Could you check a few things on this model? Use its own coordinates, in mm. A direction names the side the tool comes from. Coordinates: 2 decimals unless noted, no trailing zeros. Loops run counter-clockwise (first coordinate to the right, second up) from the corner with the lowest first, then second, coordinate; pieces in that order, holes last. Notation, with made-up numbers: (89, 2) -> (98, 2) arc R17 cw to (98, 18) -> close; hole circle Ø3 at (32.5, 65.25). An arc over 180 degrees is marked (long way). One line per question, with ' | ' between items.
Autodesk Inventor part; units mm, degrees
ref_plane "YZ Plane" through (0, 0, 0) normal (1, 0, 0) x (0, 1, 0)
ref_plane "XZ Plane" through (0, 0, 0) normal (0, 1, 0) x (-1, 0, 0)
ref_plane "XY Plane" through (0, 0, 0) normal (0, 0, 1) x (1, 0, 0)
sketch "Sketch1" plane through (0, 0, 0) normal (0, 0, 1) x (1, 0, 0)
  line L0 (-48, 48) -> (48, 48) construction
  line L1 (48, 48) -> (48, -48) construction
  line L2 (48, -48) -> (-48, -48) construction
  line L3 (-48, -48) -> (-48, 48) construction
  circle A0 centre (-45, 45) radius 2.25
  circle A1 centre (45, 45) radius 2.25
  line L4 (45, 45) -> (-45, 45) construction
  line L5 (-45, 45) -> (-45, -45) construction
  line L6 (-45, -45) -> (45, -45) construction
  line L7 (45, -45) -> (45, 45) construction
  circle A2 centre (45, -45) radius 2.25
  circle A3 centre (-45, -45) radius 2.25
  line L8 (-50.5, -50.5) -> (-42, -50.5)
  line L9 (-42, -50.5) -> (-42, -42)
  line L10 (-42, -42) -> (-50.5, -42)
  line L11 (-50.5, -42) -> (-50.5, -50.5)
  line L12 (0, 0) -> (-48, -48) construction
  line L13 (-33, 26.5) -> (33, 26.5)
  line L14 (33, 26.5) -> (33, -26.5)
  line L15 (33, -26.5) -> (-33, -26.5)
  line L16 (-33, -26.5) -> (-33, 26.5)
  line L17 (-2.4749, 2.4749) -> (2.4749, -2.4749)
  line L18 (2.4749, -2.4749) -> (-42.5251, -47.4749)
  line L19 (-42.5251, -47.4749) -> (-47.4749, -42.5251)
  line L20 (-47.4749, -42.5251) -> (-2.4749, 2.4749)
  line L21 (0, 0) -> (-45, -45) construction
  line L22 (31, 24.5) -> (-31, 24.5)
  line L23 (-31, 24.5) -> (-31, -24.5)
  line L24 (-31, -24.5) -> (31, -24.5)
  line L25 (31, -24.5) -> (31, 24.5)
  point P0 (0, 48)
  point P1 (48, 0)
  point P2 (33, 0)
  point P3 (0, 26.5)
  dimension "d0" = 96
  dimension "d1" = 96
  dimension "d2" = 4.5
  dimension "d3" = 4.5
  dimension "d4" = 3
  dimension "d5" = 4.5
  dimension "d6" = 4.5
  dimension "d9" = 3
  dimension "d10" = 3
  dimension "d11" = 66
  dimension "d12" = 53
  dimension "d13" = 7
  dimension "d14" = 0
  dimension "d23" = 5.5
  dimension "d24" = 5.5
  dimension "d25" = 2
extrude "Extrusion1" add sketch "Sketch1" along normal blind 1.5 contours L20 L24 L18 L15 | L15 L16 L13 L14 L18 L24 L25 L22 L23 L20 | L24 L23 L22 L25 L18 L17 L20 | L20 L17 L18 L24
extrude "Extrusion2" add sketch "Sketch1" along normal blind 1.5 contours A3 L19 | A3 L19 L20 L10 L9 L18 | A3 L19 L18 L9 L8 L11 L10 L20 | L20 L15 L18 L9 L10 | L20 L24 L18 L15 | L20 L17 L18 L24 picked at (-45.2318, -44.2867)
extrude "Extrusion3" cut sketch "Sketch1" along normal blind 10 contours A3 L19 | L19 A3
mirror "Mirror1" about plane through (0, 0, 0) normal (1, 0, 0) of "Extrusion2", "Extrusion3"
mirror "Mirror2" about plane through (0, 0, 0) normal (0, 1, 0) of "Extrusion2", "Extrusion3", "Mirror1"
extrude "Extrusion4" cut sketch "Sketch1" along normal blind 10 contours L24 L23 L22 L25 L18 L17 L20 | L20 L17 L18 L24
fillet "Fillet3" radius 3 4 edges at (31.4497, -26.5, 0.75) (31.4497, 26.5, 0.75) (-31.4497, 26.5, 0.75) (-31.4497, -26.5, 0.75)
fillet "Fillet4" radius 10 4 edges at (-21.5503, -26.5, 0.75) (21.5503, -26.5, 0.75) (21.5503, 26.5, 0.75) (-21.5503, 26.5, 0.75)
properties part number "BattHolder"
Q1. Imagine slicing it at C-C on x = 45. Write out the boundary of the cut face in (y, z), plus the area to 3 significant figures.
Values follow:
outline: (-50.5, 0) -> (-47.25, 0) -> (-47.25, 1.5) -> (-50.5, 1.5) -> close; (-42.75, 0) -> (-40.05, 0) -> (-40.05, 1.5) -> (-42.75, 1.5) -> close; (40.05, 0) -> (42.75, 0) -> (42.75, 1.5) -> (40.05, 1.5) -> close; (47.25, 0) -> (50.5, 0) -> (50.5, 1.5) -> (47.25, 1.5) -> close | area: 17.8 mm2
Q2. We'd pull the mould along X, two halves only. Please class faces 4 (the face through (21.286, -27.282, 0.76)), 5 (the face through (-40.5, -35.55, 0.74)), 6 (the face through (-21.286, 27.282, 0.76)), 7 (the face through (0, 26, 1.5)): released by +X, released by -X, zero draft, split by the parting line, or undercut.
Values follow:
face 4: undercut | face 5: released by -X | face 6: undercut | face 7: zero draft
Q3. Imagine slicing it at A-A on y = 2.5. Write out the boundary of the cut face in (x, z).
Values follow:
outline: (-33, 0) -> (-31, 0) -> (-31, 1.5) -> (-33, 1.5) -> close; (31, 0) -> (33, 0) -> (33, 1.5) -> (31, 1.5) -> close
Q4. For pin 1 (0.8 mm diameter, centred on x = -7.5, z = 0.5, fed in from -Y); pin 2 (0.8 mm diameter, centred on x = -1, z = 0.5, fed in from +Y), each with a flat end and sliding along its axis, tell me the tip position at first contact or that it passes through.
Values follow:
pin 1: stops at y = -26.5 | pin 2: stops at y = 26.5
Q5. For faces 1 (the face through (-40.32, 35.37, 0.74)), 2 (the face through (40.32, -35.37, 0.74)), 3 (the face through (-33.36, 38.31, 0.74)), which set-ups out of +Z, -Z, +X, -X, +Y, -Y let a thin tool reach every point of the face, with its end or its side?
Values follow:
face 1: +Z, -Z, -X | face 2: +Z, -Z, +X | face 3: +Z, -Z, +Y
Q6. Please list where these lines run through material, in increasing order: L1, parallel to Y at x = 10, z = 0.8; L2, parallel to Y at x = -45, z = 1.1. Write a range as [from, to].
Values follow:
L1: y = [-26.5, -24.5], [24.5, 26.5] | L2: y = [-50.5, -47.25], [-42.75, -40.05], [40.05, 42.75], [47.25, 50.5]
Q7. Imagine slicing it at B-B on x = -5. Write out the boundary of the cut face in (y, z), plus the area to 3 significant figures.
Values follow:
outline: (-26.5, 0) -> (-24.5, 0) -> (-24.5, 1.5) -> (-26.5, 1.5) -> close; (24.5, 0) -> (26.5, 0) -> (26.5, 1.5) -> (24.5, 1.5) -> close | area: 6.00 mm2
